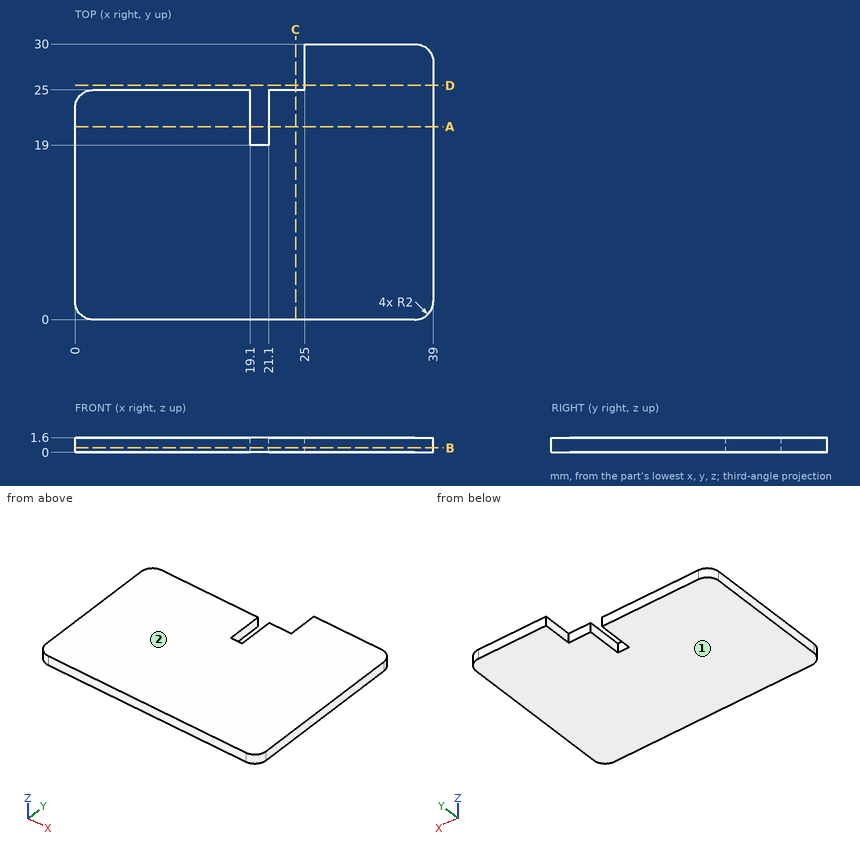
The figure shows three views and two pictorial views of one solid part (mm, origin at its lowest corner). Answer the questions. Give positions to 0.01 mm unless a question says otherwise; leave off trailing zeros. Write each loop counter-clockwise with the first axis right and the second up, starting at its lowest first coordinate (ties: lowest second). Pieces come first, ordered by that corner, then holes. Notation, with made-up numbers: M 64.25,25 L 95.25,25 A17 ccw 95.25,46 Z; hole C -3.5,-19.5 d1. An arc over 180 degrees is marked long. One line per item, written item: value. Start each with the question number.
(1) Find the intervals of material crossed by line 1 (X direction, y = 20, z = 1.2); line 2 (Y direction, x = 2.5, z = 0.45); line 3 (X direction, y = 25.5, z = 0.95), in increasing order.
(2) Find section C-C (x = 24). Determine the outline of the cut face in (y, z).
(3) A flat-ended cylindrical pin translates along its axis: pin 1 Ø0.8 at (x, z) = (24, 1) entering from +Y. Find the tip coordinate at first contact, or state that the pin passes through.
(4) Find section D-D (y = 25.5). Determine the outline of the cut face in (x, z).
(5) Find section B-B (z = 0.5). Determine the outline of the cut face in (x, y).
(6) Find section A-A (y = 21). Determine the outline of the cut face in (x, z).
(7) Determine the mould class of the marked faces 1 and 2 for opening direction Z: pulls with the +Z half, pulls with the -Z half, needs draft (parallel to the pull), parting line crosses it, or undercut.
Results below:
1. line 1: x = 0 to 19.1, 21.1 to 39
1. line 2: y = 0 to 25
1. line 3: x = 25 to 39
2. outline: M 0,0 L 25,0 L 25,1.6 L 0,1.6 Z
3. pin 1: stops at y = 25
4. outline: M 25,0 L 39,0 L 39,1.6 L 25,1.6 Z
5. outline: M 0,2 A2 ccw 2,0 L 37,0 A2 ccw 39,2 L 39,28 A2 ccw 37,30 L 25,30 L 25,25 L 21.1,25 L 21.1,19 L 19.1,19 L 19.1,25 L 2,25 A2 ccw 0,23 Z
6. outline: M 0,0 L 19.1,0 L 19.1,1.6 L 0,1.6 Z; M 21.1,0 L 39,0 L 39,1.6 L 21.1,1.6 Z
7. face 1: pulls with the -Z half
7. face 2: pulls with the +Z half
